Part print with two shaded views. Sizes in mm from the minimum x, y, z corner. A direction names the side the tool comes from. Round coordinates to 2 decimals unless told otherwise and drop trailing zeros. Loops run counter-clockwise (first coordinate to the right, second up) from the corner with the lowest first, then second, coordinate; pieces in that order, holes last. Notation, with made-up numbers: (57, 11.5) - (92, 11.5) arc R19 cw to (92, 28.5) - close; hole circle Ø9 at (-37.5, 34). An arc over 180 degrees is marked (long way). Write each question's results on one line, items separated by ' | '. Start each with the question number.
(1) Flat gauge pins, fed straight in: P1, Ø10, axis at x = 16, z = 17.5, coming from the -Y side; P2, Ø1.5, axis at x = 19, y = 25.5, coming from the -Z side; P3, Ø3, axis at x = 85.5, y = 21.5, coming from the -Z side. Where does each tip first touch, or does it go through?
(2) Tool access for the marked faces 4 and 5: list every direction of +Z, -Z, +X, -X, +Y, -Y with a clear straight run to the whole face (end or side of a thin tool).
(3) Cut at A-A, the plane x = 44.5. List the corners of the cut face in (y, z) (1 decimal), then the cut area to 3 significant figures.
(4) Cut at C-C, the plane y = 48.5. List the corners of the cut face in (x, z), then the cut area to 3 significant figures.
(5) Drill centre lines: L1, parallel to Y at x = 28.5, z = 42.5; L2, parallel to X at y = 48.5, z = 57 (1 decimal); L3, parallel to X at y = 16, z = 29.5 (1 decimal). Where is each one in solid material? Low to high.
(6) Cut at D-D, the plane x = 29. List the corners of the cut face in (y, z), then the cut area to 3 significant figures.
(7) Mould opens along X. For the marked faces 1, 2 and 3 say: released by +X, released by -X, zero draft, split by the parting line, or undercut.
(8) Cut at B-B, the plane z = 61. List the corners of the cut face in (x, y) (1 decimal).
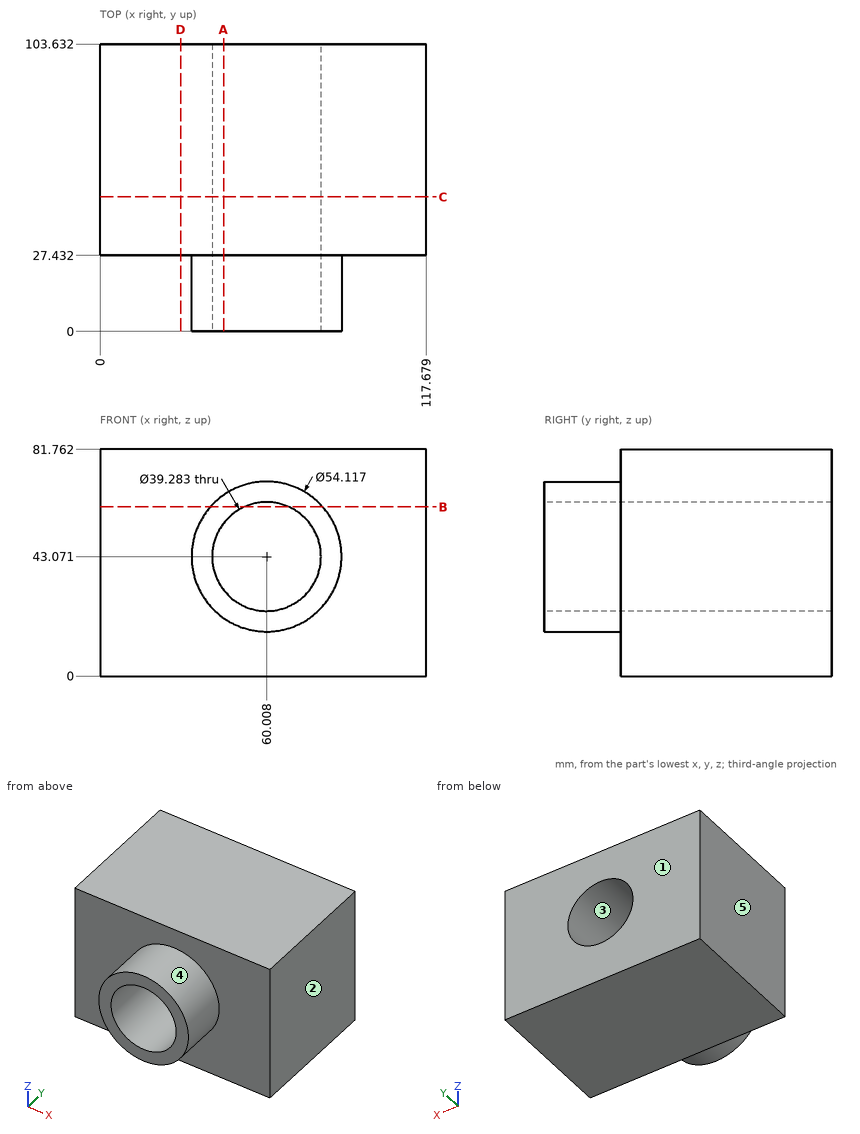
A:
1) P1: y = 27.43 | P2: through | P3: z = 30.56
2) face 4: -Y | face 5: +Z, -Z, -X, +Y, -Y
3) outline: (0, 20.9) - (27.4, 20.9) - (27.4, 0) - (103.6, 0) - (103.6, 31) - (0, 31) - close; (0, 55.1) - (103.6, 55.1) - (103.6, 81.8) - (27.4, 81.8) - (27.4, 65.2) - (0, 65.2) - close | area: 4,950 mm2
4) outline: (0, 0) - (117.68, 0) - (117.68, 81.76) - (0, 81.76) - close; hole circle Ø39.28 at (60.01, 43.07) | area: 8,410 mm2
5) L1: 27.43 to 103.63 | L2: 0 to 46.2, 73.9 to 117.7 | L3: 36.6 to 45.8, 74.2 to 83.4
6) outline: (27.43, 0) - (103.63, 0) - (103.63, 81.76) - (27.43, 81.76) - close | area: 6,230 mm2
7) face 1: zero draft | face 2: released by +X | face 3: undercut
8) outline: (0, 27.4) - (39.7, 27.4) - (39.7, 0) - (52, 0) - (52, 103.6) - (0, 103.6) - close; (68, 0) - (80.3, 0) - (80.3, 27.4) - (117.7, 27.4) - (117.7, 103.6) - (68, 103.6) - close
